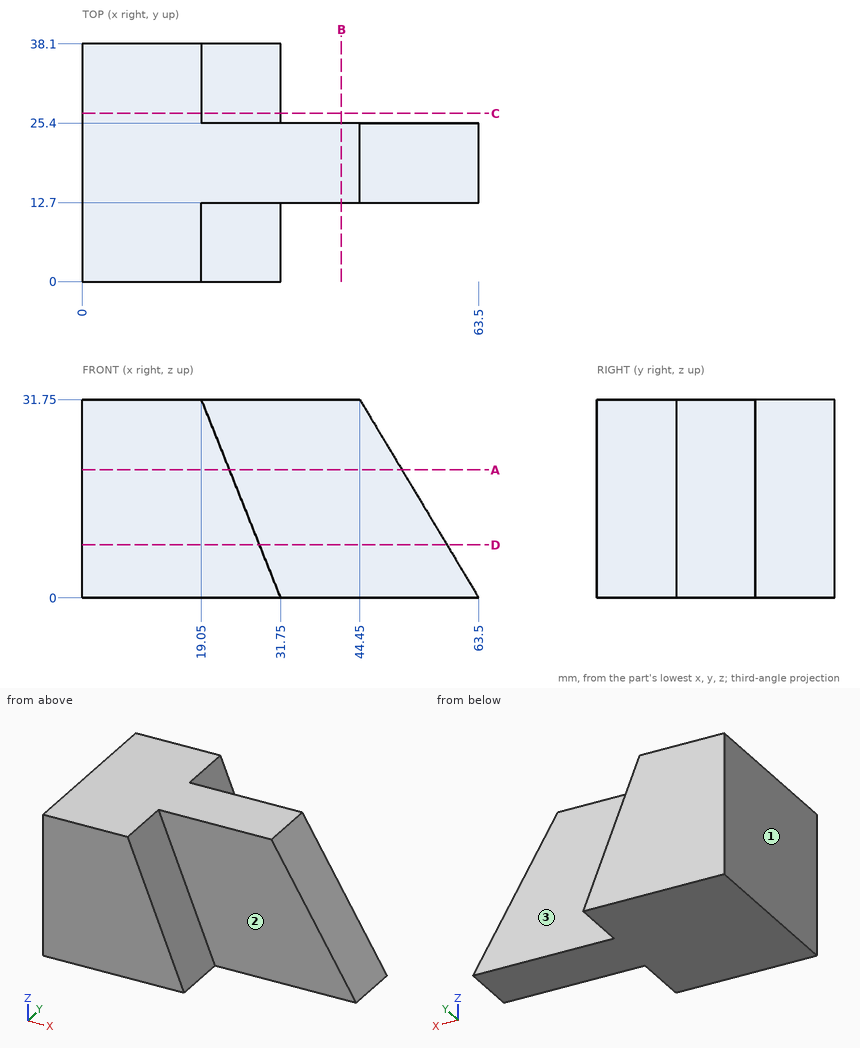
Verification items for this drawing (mm, ordinates from the low corner). A direction names the side the tool comes from. Give positions to 0.01 mm unless a question says otherwise; leave off trailing zeros. Order: outer loops, then holes, each group sorted by start corner. A loop starts at its lowest first (then second) coordinate and runs counter-clockwise, first axis right, second up.
1) Cross-section at B-B (x = 41.5). Record the boundary of the cut face in (y, z), then the cut area to 3 significant figures.
Results are:
outline: (12.7, 0) - (25.4, 0) - (25.4, 31.75) - (12.7, 31.75) - close
area: 403 mm2
2) Cross-section at D-D (z = 8.5). Record the boundary of the cut face in (x, y).
Results are:
outline: (0, 0) - (28.35, 0) - (28.35, 12.7) - (58.4, 12.7) - (58.4, 25.4) - (28.35, 25.4) - (28.35, 38.1) - (0, 38.1) - close
3) Gauge pin test, flat ends, axial feed: pin 1 (16 mm diameter, centred on x = 45.5, z = 21.5, fed in from +Y); pin 2 (10 mm diameter, centred on y = 33.5, z = 16, fed in from +X); pin 3 (12 mm diameter, centred on y = 18.5, z = 7.5, fed in from +X). Record the tip position at first contact, or that the pin passes through.
Results are:
pin 1: stops at y = 25.4
pin 2: stops at x = 27.35
pin 3: stops at x = 62.6
4) Tool access check on the marked faces 1, 2 and 3. Record the directions out of +Z, -Z, +X, -X, +Y, -Y that give a thin tool (end or side, any length) a straight path to the whole face; none if there is none.
Results are:
face 1: +Z, -Z, -X, +Y, -Y
face 2: +Z, +X, -Y
face 3: +Z, +X, +Y
5) Cross-section at A-A (z = 20.5). Record the boundary of the cut face in (x, y).
Results are:
outline: (0, 0) - (23.55, 0) - (23.55, 12.7) - (51.2, 12.7) - (51.2, 25.4) - (23.55, 25.4) - (23.55, 38.1) - (0, 38.1) - close
6) Material ranges on probe 1 along Y at (x, z) = (43, 14.5); probe 2 along X at (y, z) = (3, 23.5); probe 3 along X at (y, z) = (17.5, 28), recorded low to high.
Results are:
probe 1: y = 12.7 to 25.4
probe 2: x = 0 to 22.35
probe 3: x = 0 to 46.7
7) Cross-section at C-C (y = 27). Record the boundary of the cut face in (x, z).
Results are:
outline: (0, 0) - (31.75, 0) - (19.05, 31.75) - (0, 31.75) - close
